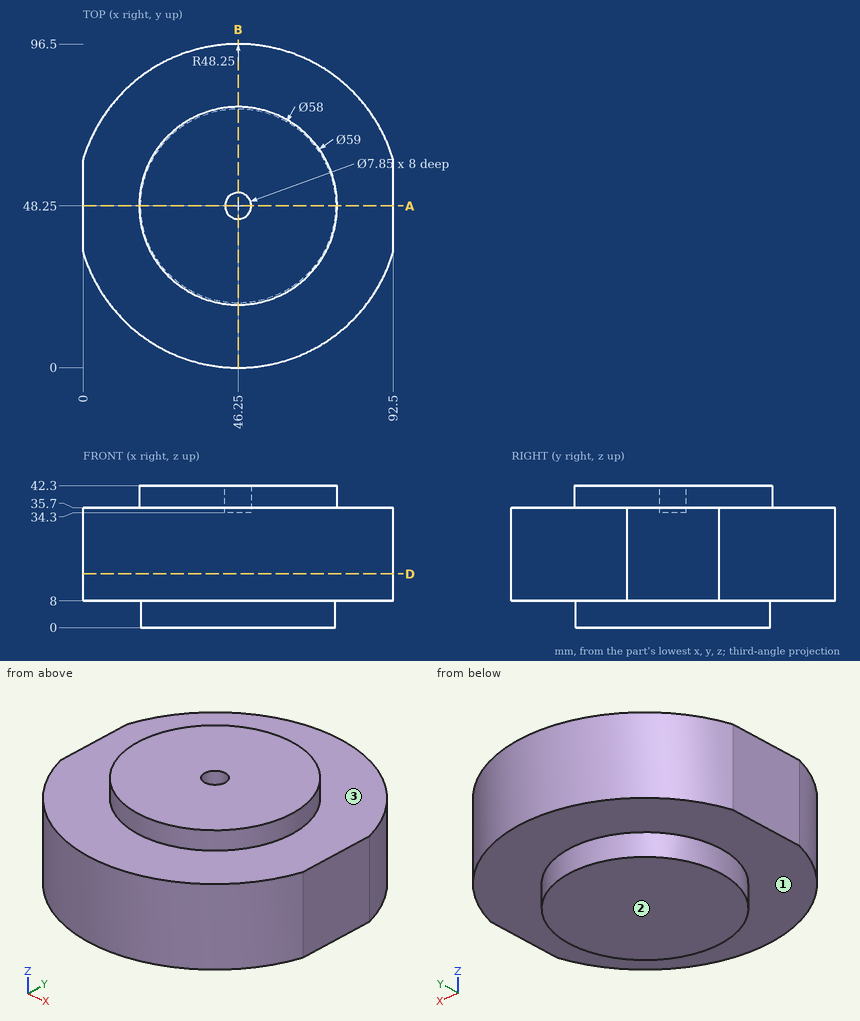
Print and shaded views of the part. All mm, measured from the part's lowest x, y and z. A direction names the side the tool comes from. Coordinates: 2 decimals unless noted, no trailing zeros. Write each loop counter-clockwise with the first axis right and the second up, starting at its lowest first coordinate (ties: lowest second). Pieces come first, ordered by that corner, then holes. Notation, with made-up numbers: M 47.5,6.5 L 99.5,6.5 A11 ccw 99.5,19.5 Z; hole C -18,-30.75 d8. An arc over 180 degrees is marked long. Return JSON: item names as keys, results as strings.
1. 3-axis set-ups, long thin cutter, end or side, ignore diameter. For the marked faces 1, 2 and 3: which of +Z, -Z, +X, -X, +Y, -Y reach the whole face in a straight line?
Determined:
{"face 1": "-Z", "face 2": "-Z, +X, -X, +Y, -Y", "face 3": "+Z"}
2. Saw through at B-B, the plane x = 46.25. Write the cut outline in (y, z) (3 decimals), then the cut area to 3 significant figures.
Determined:
{"outline": "M 0,8 L 19.25,8 L 19.25,0 L 77.25,0 L 77.25,8 L 96.5,8 L 96.5,35.7 L 77.75,35.7 L 77.75,42.3 L 52.175,42.3 L 52.175,34.3 L 44.325,34.3 L 44.325,42.3 L 18.75,42.3 L 18.75,35.7 L 0,35.7 Z", "area": "3,460 mm²"}
3. Probe L1, parallel to Y at x = 46.25, z = 38.5 (3 decimals); L2, parallel to X at y = 48, z = 39; L3, parallel to Z at x = 8.5, y = 58. List the from-to ranges inside material, lowest first.
Determined:
{"L1": "18.75 to 44.325, 52.175 to 77.75", "L2": "16.75 to 42.33, 50.17 to 75.75", "L3": "8 to 35.7"}
4. Flat gauge pins, fed straight in: pin 1 Ø6 at (x, z) = (79.5, 10.5) entering from -Y; pin 2 Ø1 at (y, z) = (75, 33.5) entering from -X (1 decimal); pin 3 Ø1.5 at (x, z) = (75, 18.5) entering from -Y (1 decimal). Where does each tip first touch, or does it go through?
Determined:
{"pin 1": "y = 10.66", "pin 2": "x = 5.8", "pin 3": "y = 9"}
5. Saw through at A-A, the plane y = 48.25. Write the cut outline in (x, z) (3 decimals), then the cut area to 3 significant figures.
Determined:
{"outline": "M 0,8 L 17.25,8 L 17.25,0 L 75.25,0 L 75.25,8 L 92.5,8 L 92.5,35.7 L 75.75,35.7 L 75.75,42.3 L 50.175,42.3 L 50.175,34.3 L 42.325,34.3 L 42.325,42.3 L 16.75,42.3 L 16.75,35.7 L 0,35.7 Z", "area": "3,350 mm²"}
6. Saw through at D-D, the plane z = 16. Write the cut outline in (x, y), then the cut area to 3 significant figures.
Determined:
{"outline": "M 0,34.5 A48.25 ccw 92.5,34.5 L 92.5,62 A48.25 ccw 0,62 Z", "area": "7,240 mm²"}
